The listing builds one solid part. Answer for the finished solid, in the listing's coordinates (mm). A direction names the side the tool comes from. Round coordinates to 2 decimals unless told otherwise and drop trailing zeros. Write each loop counter-clockwise with the first axis right and the second up, starting at its lowest first coordinate (ties: lowest second). Pieces come first, ordered by that corner, then holes.
Item 1: Find section C-C on x = 49.5. Give the vertices of the cut face in (y, z), then the cut area to 3 significant figures.
Item 2: Find section A-A on y = 0. Give the vertices of the cut face in (x, z).
Item 3: Find the intervals of material crossed by probe 1 along Z at (x, y) = (89, -13.5); probe 2 along Z at (x, y) = (-35, 0.5); probe 3 along X at (y, z) = (-20, 10), in increasing order.
Item 4: A tool of negligible diameter and unlimited length cuts with its end or side. For faces 4 (the face through (65, -12, 20)), 5 (the face through (110, 0, 10)), 6 (the face through (-52.22, 0.44, 66.56)), from which of +Z, -Z, +X, -X, +Y, -Y can it reach the whole face along a straight path? Write none if from no direction.
Item 5: For a pull along Y with two mould halves and no side action, classify faces 1 (the face through (20, 0, 10)), 2 (the face through (-63.536, -0.572, 77.876)), 3 (the face through (59, -12, 0)) as +Y half, -Y half, draft (parallel to the pull), parting line (faces both ways), or undercut.
Item 6: Each of these flat-tipped pins is pushed along its axis until it touches: pin 1 (12 mm diameter, centred on x = 34.5, y = 19, fed in from +Z); pin 2 (1 mm diameter, centred on y = -13.5, z = 74, fed in from +X); pin 3 (1 mm diameter, centred on y = 7, z = 8.5, fed in from -X); pin 4 (10 mm diameter, centred on x = 28, z = 23.5, fed in from +Y). Where does it stop, or does it pass through?
Item 7: Find section B-B on z = 16.5. Give the vertices of the cut face in (x, y), then the cut area to 3 significant figures.
Item 8: Find section D-D on y = -15.5. Give the vertices of the cut face in (x, z), then the cut area to 3 significant figures.
```python
from build123d import *

# Parameters (mm, degrees)
F1_DEPTH = 26
F3_DEPTH = 20.001
F4_R     = 10
F5_DEPTH = 70.001


with BuildPart() as f1:
    # F0 (on Front) → F1 (new body, symmetric)
    with BuildSketch(Plane.XZ):
        Polygon((-70.7106781187, 70.7106781187), (0, 0), (120, 0), (120, 20), (8.2842712475, 20), (-56.5685424949, 84.8528137424), align=None)
    extrude(amount=F1_DEPTH, both=True)

    # F2 (on face) → F3 (cut, through all)
    with BuildSketch(Plane.XY.offset(20)):
        with BuildLine():
            Line((30, -10), (100, -10))
            ThreePointArc((100, -10), (110, 0), (100, 10))
            Line((100, 10), (30, 10))
            ThreePointArc((30, 10), (20, 0), (30, -10))
        make_face()
    extrude(amount=-F3_DEPTH, mode=Mode.SUBTRACT)

    # F4 (on face) → F5 (cut, through all)
    with BuildSketch(Plane(origin=(14.1421356237, 0, 14.1421356237), x_dir=(0.7071067812, 0, -0.7071067812), z_dir=(0.7071067812, 0, 0.7071067812))):
        with Locations((-74, 0)):
            Circle(F4_R)
        with BuildLine():
            ThreePointArc((-74, -26), (-92.3847763543, -18.3847762674), (-100, 1.228e-07))
            Line((-100, 1.228e-07), (-100, -26))
            Line((-100, -26), (-74, -26))
        make_face()
        with BuildLine():
            ThreePointArc((-100, 1.228e-07), (-92.3847762674, 18.3847763543), (-74, 26))
            Line((-74, 26), (-100, 26))
            Line((-100, 26), (-100, 1.228e-07))
        make_face()
    extrude(amount=-F5_DEPTH, mode=Mode.SUBTRACT)


solid = f1.part
```
Check values:
1. outline: (-26, 0) - (-10, 0) - (-10, 20) - (-26, 20) - close; (10, 0) - (26, 0) - (26, 20) - (10, 20) - close
1. area: 640 mm2
2. outline: (-70.71, 70.71) - (-59.4, 59.4) - (-45.25, 73.54) - (-56.57, 84.85) - close; (-45.25, 45.25) - (0, 0) - (20, 0) - (20, 20) - (8.28, 20) - (-31.11, 59.4) - close; (110, 0) - (120, 0) - (120, 20) - (110, 20) - close
3. probe 1: z = 0 to 20
3. probe 2: z = 35 to 55.53
3. probe 3: x = -10 to 120
4. face 4: +Z, +X, +Y, -Y
4. face 5: +Z, -Z
4. face 6: none
5. face 1: undercut
5. face 2: parting line
5. face 3: draft
6. pin 1: stops at z = 20
6. pin 2: stops at x = -45.22
6. pin 3: stops at x = -9
6. pin 4: stops at y = 26
7. outline: (-16.5, -26) - (120, -26) - (120, 26) - (-16.5, 26) - close; hole (30, -10) - (100, -10) arc R10 ccw to (100, 10) - (30, 10) arc R10 ccw to start
7. area: 5,380 mm2
8. outline: (-67.09, 67.09) - (0, 0) - (120, 0) - (120, 20) - (8.28, 20) - (-52.94, 81.23) - close
8. area: 4,130 mm2
